For this review, take the finished solid that the model builds, in its own axes (mm). Face numbers are marked on the shaded views. A direction names the side the tool comes from. Give positions to 0.01 mm unless a question says otherwise; leave off trailing zeros. Write each loop counter-clockwise with the first axis right and the second up, starting at its lowest first coordinate (ties: lowest second). Pieces come first, ordered by that corner, then holes. Notation, with made-up numbers: (38.25, 49) -> (88.25, 49) arc R24 ccw to (88.25, 60) -> close; hole circle Ø3 at (17.25, 60.25). An arc over 180 degrees is marked (long way). Return JSON: item names as keys, results as strings.
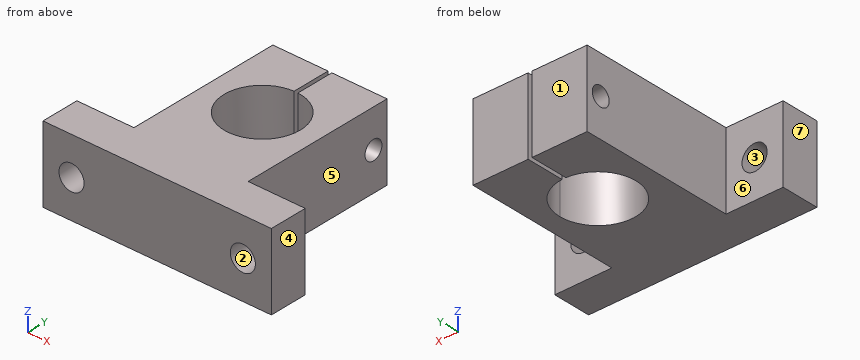
from build123d import *

# Parameters (mm, degrees)
SKETCH1_R           = 10
BOSS_EXTRUDE1_DEPTH = 20
SKETCH3_W           = 1
SKETCH3_H           = 10.850896804
CUT_EXTRUDE1_DEPTH  = 59
SKETCH2_R           = 2.5
CUT_EXTRUDE3_DEPTH  = 31
SKETCH5_R           = 3.3
CUT_EXTRUDE5_DEPTH  = 22


with BuildPart() as part:
    # Sketch1 → Boss-Extrude1 (new body)
    with BuildSketch(Plane.XY):
        Polygon((-30, 0), (30, 0), (30, 10), (15, 10), (15, 51), (-15, 51), (-15, 10), (-30, 10), align=None)
        with Locations((0, 31)):
            Circle(SKETCH1_R, mode=Mode.SUBTRACT)
    extrude(amount=BOSS_EXTRUDE1_DEPTH)

    # Sketch3 → Cut-Extrude1 (cut)
    with BuildSketch(Plane.XY.offset(20)):
        with Locations((0, 45.574551598)):
            Rectangle(SKETCH3_W, SKETCH3_H)
    extrude(amount=-CUT_EXTRUDE1_DEPTH, mode=Mode.SUBTRACT)

    # Sketch2 → Cut-Extrude3 (cut)
    with BuildSketch(Plane(origin=(15, 0, 0), x_dir=(0, 0, -1), z_dir=(1, 0, 0))):
        with Locations((-10, 47)):
            Circle(SKETCH2_R)
    extrude(amount=-CUT_EXTRUDE3_DEPTH, mode=Mode.SUBTRACT)

    # Sketch5 → Cut-Extrude5 (cut)
    with BuildSketch(Plane(origin=(0, 10, 0), x_dir=(1, 0, 0), z_dir=(0, 1, 0))):
        with Locations((22.5, -10)):
            Circle(SKETCH5_R)
        with Locations((-22.5, -10)):
            Circle(SKETCH5_R)
    extrude(amount=-CUT_EXTRUDE5_DEPTH, mode=Mode.SUBTRACT)


solid = part.part
1. Add section B-B, the plane y = 47. State the section outline as (x, z) points, plus the area to 3 significant figures.
Results found:
{"outline": "(-15, 0) -> (-0.5, 0) -> (-0.5, 7.5) -> (-15, 7.5) -> close; (-15, 12.5) -> (-0.5, 12.5) -> (-0.5, 20) -> (-15, 20) -> close; (0.5, 0) -> (15, 0) -> (15, 7.5) -> (0.5, 7.5) -> close; (0.5, 12.5) -> (15, 12.5) -> (15, 20) -> (0.5, 20) -> close", "area": "435 mm²"}
2. Add section C-C, the plane x = -22.5. State the section outline as (y, z) points, plus the area to 3 significant figures.
Results found:
{"outline": "(0, 0) -> (10, 0) -> (10, 6.7) -> (0, 6.7) -> close; (0, 13.3) -> (10, 13.3) -> (10, 20) -> (0, 20) -> close", "area": "134 mm²"}
3. For pin 1 (4 mm diameter, centred on y = 45, z = 13.5, fed in from -X); pin 2 (3 mm diameter, centred on y = 47, z = 7, fed in from +X); pin 3 (6 mm diameter, centred on x = 6.5, y = 22.5, fed in from -Z); pin 4 (7.5 mm diameter, centred on x = 22.5, z = 11.5, fed in from +Y), all flat-tipped, find the tip position at first contact; note any pin that passes through.
Results found:
{"pin 1": "stops at x = -15", "pin 2": "stops at x = 15", "pin 3": "stops at z = 0", "pin 4": "stops at y = 10"}
4. For the marked faces 5, 6 and 7, list the 3-axis set-ups (+Z, -Z, +X, -X, +Y, -Y) from which the entire face can be reached by the end or side of a thin tool; tool diameter is ignored.
Results found:
{"face 5": "+Z, -Z, +X, +Y", "face 6": "+Z, -Z, -X, +Y", "face 7": "+Z, -Z, -X, +Y, -Y"}
5. Add section A-A, the plane z = 10. State the section outline as (x, y) points.
Results found:
{"outline": "(-30, 0) -> (-25.8, 0) -> (-25.8, 10) -> (-30, 10) -> close; (-19.2, 0) -> (19.2, 0) -> (19.2, 10) -> (15, 10) -> (15, 44.5) -> (0.5, 44.5) -> (0.5, 40.99) arc R10 cw (long way) to (-0.5, 40.99) -> (-0.5, 44.5) -> (-15, 44.5) -> (-15, 10) -> (-19.2, 10) -> close; (-15, 49.5) -> (-0.5, 49.5) -> (-0.5, 51) -> (-15, 51) -> close; (0.5, 49.5) -> (15, 49.5) -> (15, 51) -> (0.5, 51) -> close; (25.8, 0) -> (30, 0) -> (30, 10) -> (25.8, 10) -> close"}
6. The part is to be moulded in two halves that separate along X. For the marked faces 1, 2, 3 and 4, say which applies: +X half, -X half, draft (parallel to the pull), parting line (faces both ways), or undercut.
Results found:
{"face 1": "draft", "face 2": "undercut", "face 3": "undercut", "face 4": "+X half"}
7. To check wall thickness, follow probe 1 along X at (y, z) = (45.5, 18.75); probe 2 along X at (y, z) = (2.75, 10); probe 3 along Z at (x, y) = (-22.5, 2.25). State the ranges of each line that lie inside material, in increasing order.
Results found:
{"probe 1": "x = -15 to -0.5, 0.5 to 15", "probe 2": "x = -30 to -25.8, -19.2 to 19.2, 25.8 to 30", "probe 3": "z = 0 to 6.7, 13.3 to 20"}
8. Add section D-D, the plane y = 39. State the section outline as (x, z) points.
Results found:
{"outline": "(-15, 0) -> (-6, 0) -> (-6, 20) -> (-15, 20) -> close; (6, 0) -> (15, 0) -> (15, 20) -> (6, 20) -> close"}
